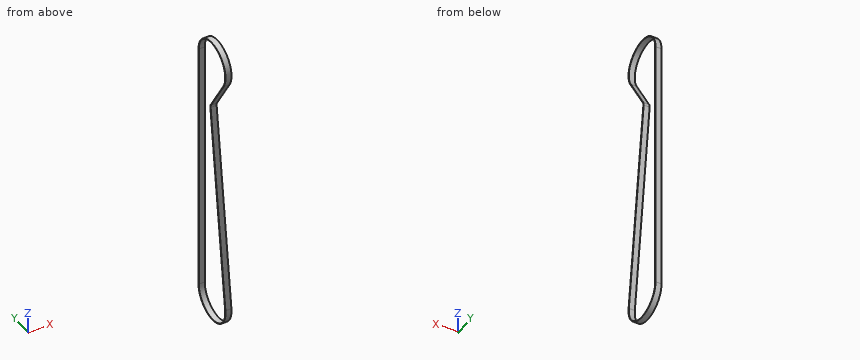
Autodesk Inventor part; units mm, degrees
ref_plane "YZ Plane" through (0, 0, 0) normal (1, 0, 0) x (0, 1, 0)
ref_plane "XZ Plane" through (0, 0, 0) normal (0, 1, 0) x (-1, 0, 0)
ref_plane "XY Plane" through (0, 0, 0) normal (0, 0, 1) x (1, 0, 0)
sketch "スケッチ1" plane through (0, 0, 0) normal (1, 0, 0) x (0, 1, 0)
  arc A0 (38.1972, 0) -> (-32.7626, -19.6376) centre (0, 0) ccw
  arc A1 (-37.9221, -435.4244) -> (38.1972, -440) centre (0, -440) ccw
  arc A2 (4.3584, -85.0085) -> (3.2212, -79.6717) centre (-4, -84) ccw
  line L0 (3.2212, -79.6717) -> (-32.7626, -19.6376)
  line L1 (38.1972, -440) -> (38.1972, 0)
  line L2 (4.3584, -85.0085) -> (-37.9221, -435.4244)
  arc A3 (38.6162, 0) -> (-33.122, -19.853) centre (0, 0) ccw
  line L3 (-33.122, -19.853) -> (2.8618, -79.8871)
  arc A4 (3.9424, -84.9583) -> (2.8618, -79.8871) centre (-4, -84) ccw
  line L4 (3.9424, -84.9583) -> (-38.3381, -435.3742)
  arc A5 (-38.3381, -435.3742) -> (38.6162, -440) centre (0, -440) ccw
  line L5 (38.6162, -440) -> (38.6162, 0)
  arc A6 (37.8162, 0) -> (-32.4358, -19.4417) centre (0, 0) ccw
  line L6 (-32.4358, -19.4417) -> (3.548, -79.4758)
  arc A7 (4.7366, -85.0541) -> (3.548, -79.4758) centre (-4, -84) ccw
  line L7 (4.7366, -85.0541) -> (-37.5439, -435.47)
  arc A8 (-37.5439, -435.47) -> (37.8162, -440) centre (0, -440) ccw
  line L8 (37.8162, -440) -> (37.8162, 0)
  dimension "d0" = 76.3944
  dimension "d1" = 76.3944
  dimension "d2" = 440
  dimension "d24" = 0.419
  dimension "d25" = 8
  dimension "d26" = 84
  dimension "d27" = 0.8
  dimension "d30" = 4
extrude "押し出し1" add sketch "スケッチ1" along normal mid plane 10 contours L1 A1 L2 A2 L0 A0 | L5 A5 L4 A4 L3 A3
properties part number "belt_1" material "ゴム"
Geometry check sheet. Reference: the model listing, model coordinates, mm. Give positions to 0.01 mm unless a question says otherwise; leave off trailing zeros. Write each loop counter-clockwise with the first axis right and the second up, starting at its lowest first coordinate (ties: lowest second). Pieces come first, ordered by that corner, then holes.
1) Section check A-A, the plane x = -0.5. Record the boundary of the cut face in (y, z).
2) Section check C-C, the plane y = -12. Record the boundary of the cut face in (x, z).
3) Gauge pin test, flat ends, axial feed: pin 1 (6 mm diameter, centred on x = -3, z = -114.5, fed in from -Y); pin 2 (1 mm diameter, centred on x = -0.5, y = 15.5, fed in from -Z); pin 3 (2 mm diameter, centred on x = 1, y = -21, fed in from -Z); pin 4 (5 mm diameter, centred on y = -7.5, z = -209.5, fed in from +X). Record the tip position at first contact, or that the pin passes through.
4) Section check B-B, the plane z = -445.5. Record the boundary of the cut face in (x, y).
5) Material ranges on L1, parallel to Y at x = 3.25, z = -439; L2, parallel to Y at x = -2.75, z = 2.5; L3, parallel to Z at x = 2, y = 24.5, recorded low to high.
6) Section check D-D, the plane z = -225. Record the boundary of the cut face in (x, y).
Computed:
1. outline: (-38.34, -435.37) arc R38.62 ccw (long way) to (38.62, -440) - (38.62, 0) arc R38.62 ccw (long way) to (-33.12, -19.85) - (2.86, -79.89) arc R8 cw to (3.94, -84.96) - close; hole (-37.54, -435.47) arc R37.82 ccw (long way) to (37.82, -440) - (37.82, 0) arc R37.82 ccw (long way) to (-32.44, -19.44) - (3.55, -79.48) arc R8.8 cw to (4.74, -85.05) - close
2. outline: (-5, -476.7) - (5, -476.7) - (5, -475.86) - (-5, -475.86) - close; (-5, -223.77) - (5, -223.77) - (5, -217.09) - (-5, -217.09) - close; (-5, -55.09) - (5, -55.09) - (5, -53.54) - (-5, -53.54) - close; (-5, 35.86) - (5, 35.86) - (5, 36.7) - (-5, 36.7) - close
3. pin 1: stops at y = 0.02
3. pin 2: stops at z = -475.58
3. pin 3: stops at z = -473.03
3. pin 4: passes through
4. outline: (-5, -38.22) - (5, -38.22) - (5, -37.41) - (-5, -37.41) - close; (-5, 37.41) - (5, 37.41) - (5, 38.22) - (-5, 38.22) - close
5. L1: y = -38.6 to -37.8, 37.82 to 38.62
5. L2: y = -38.54 to -37.73, 37.73 to 38.54
5. L3: z = -469.85 to -468.81, 28.81 to 29.85
6. outline: (-5, -12.95) - (5, -12.95) - (5, -12.15) - (-5, -12.15) - close; (-5, 37.82) - (5, 37.82) - (5, 38.62) - (-5, 38.62) - close
